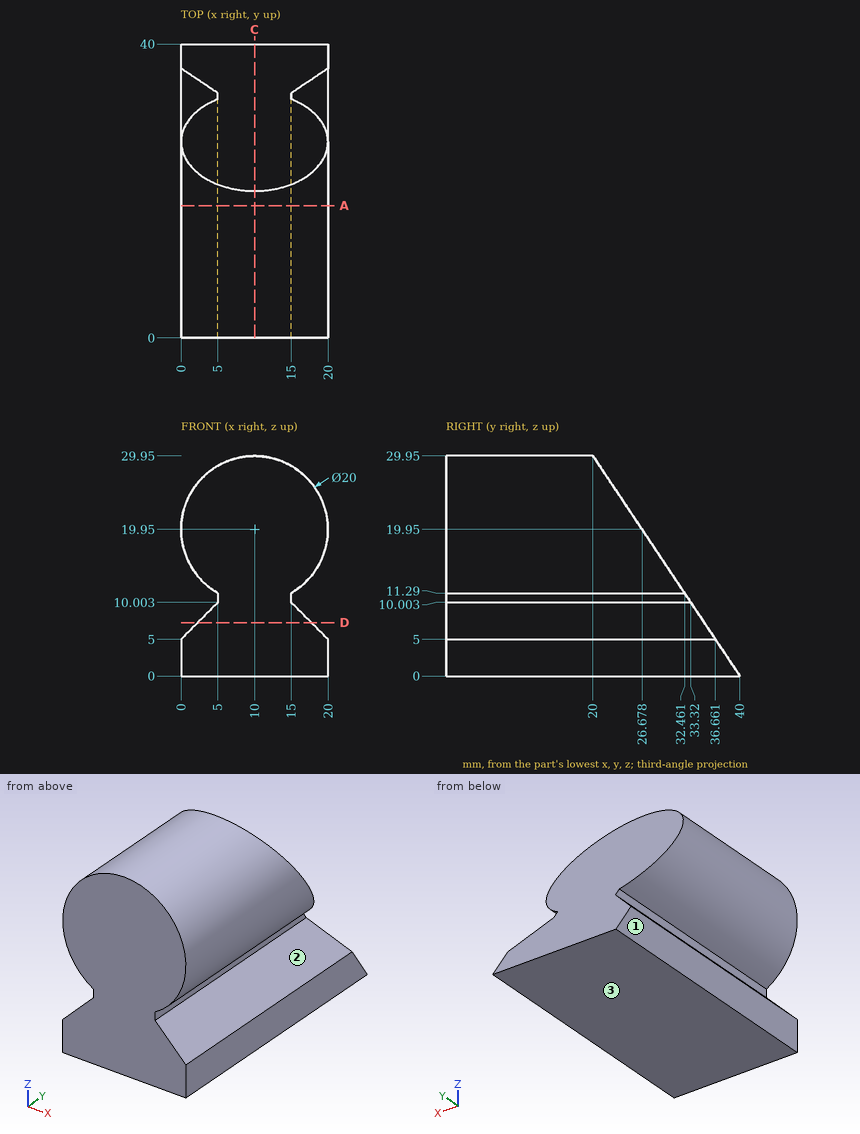
Can you work these out from the drawing? Everything is in mm from the part's minimum corner. Coordinates: 2 decimals unless noted, no trailing zeros. Write each loop counter-clockwise with the first axis right and the second up, starting at its lowest first coordinate (ties: lowest second). Pieces come first, ordered by that corner, then holes. Notation, with made-up numbers: (54, 59.5) -> (108, 59.5) arc R7 cw to (108, 63.5) -> close; hole circle Ø5 at (19.25, 29.25). An arc over 180 degrees is marked (long way). Write item = value, one per line.
(1) Thinking about a two-plate mould opening in Z: for the marked faces 1, 2 and 3, which applies, +Z half, -Z half, draft (parallel to the pull), parting line (faces both ways), or undercut?
Verdict:
face_1 = draft
face_2 = undercut
face_3 = -Z half
(2) If I drill on probe 1 along Z at (x, y) = (18, 28); probe 2 along Z at (x, y) = (3.5, 14); probe 3 along Y at (x, z) = (4, 7.5), over which ranges is the centre line in solid material (lowest first)?
Verdict:
probe_1 = 0 to 7, 13.95 to 17.97
probe_2 = 0 to 8.5, 12.35 to 27.55
probe_3 = 0 to 34.99
(3) Imagine slicing it at C-C (x = 10). Please give me the cut outline in (y, z).
Verdict:
outline = (0, 0) -> (40, 0) -> (20, 29.95) -> (0, 29.95) -> close
(4) For pin 1 (2 mm diameter, centred on y = 5, z = 7.5, fed in from -X); pin 2 (2 mm diameter, centred on y = 8, z = 15.5, fed in from +X); pin 3 (8 mm diameter, centred on x = 8.5, z = 26, fed in from +Y); pin 4 (1 mm diameter, centred on y = 32.5, z = 14, fed in from +X), each with a flat end and sliding along its axis, tell me the tip position at first contact or that it passes through.
Verdict:
pin_1 = 1.5
pin_2 = 19.39
pin_3 = 25.31
pin_4 = through
(5) Imagine slicing it at D-D (z = 7.25). Please give me the cut outline in (x, y).
Verdict:
outline = (2.25, 0) -> (17.75, 0) -> (17.75, 35.16) -> (2.25, 35.16) -> close
(6) Imagine slicing it at A-A (y = 18). Please give me the cut outline in (x, z).
Verdict:
outline = (0, 0) -> (20, 0) -> (20, 5) -> (15, 10) -> (15, 11.29) arc R10 ccw (long way) to (5, 11.29) -> (5, 10) -> (0, 5) -> close
